```python
from build123d import *

# Parameters (mm, degrees)
F0_R     = 1.5
F1_DEPTH = 20
F2_W     = 3
F2_H     = 10
F3_DEPTH = 12


with BuildPart() as f1:
    # F0 (on Top) → F1 (new body)
    with BuildSketch(Plane.XY):
        with BuildLine():
            ThreePointArc((15, 2), (14.12132, 4.12132), (12, 5))
            Line((12, 5), (-12, 5))
            ThreePointArc((-12, 5), (-14.12132, 4.12132), (-15, 2))
            Line((-15, 2), (-15, -2))
            ThreePointArc((-15, -2), (-14.12132, -4.12132), (-12, -5))
            Line((-12, -5), (12, -5))
            ThreePointArc((12, -5), (14.12132, -4.12132), (15, -2))
            Line((15, -2), (15, 2))
        make_face()
        with Locations((-10, 0)):
            Circle(F0_R, mode=Mode.SUBTRACT)
        with Locations((10, 0)):
            Circle(F0_R, mode=Mode.SUBTRACT)
    extrude(amount=F1_DEPTH)

    # F2 (on face) → F3 (cut)
    with BuildSketch(Plane(origin=(0, 0, 0), x_dir=(1, 0, 0), z_dir=(0, 0, -1))):
        Rectangle(F2_W, F2_H)
    extrude(amount=-F3_DEPTH, mode=Mode.SUBTRACT)

    # F4: F1 across face


with BuildPart() as f1_1:
    add(f1.part)
    add(f1.part.mirror(Plane.XY.offset(20)))


solid = f1_1.part
```
For this review, take the finished solid that the model builds, in its own axes (mm). A direction names the side the tool comes from. Coordinates: 2 decimals unless noted, no trailing zeros. Order: outer loops, then holes, each group sorted by start corner. A loop starts at its lowest first (then second) coordinate and runs counter-clockwise, first axis right, second up. Notation, with made-up numbers: (31, 2.25) -> (90, 2.25) arc R7 cw to (90, 12.25) -> close; hole circle Ø7 at (-22, 21). An arc over 180 degrees is marked (long way). Use CSV: the item, a comma, the result in double quotes. Start each with the question number.
Item 1: We need section B-B, the plane x = -10. Give the boundary of the cut face in (y, z).
Item 2: Insertion check: pin 1 (3.5 mm diameter, centred on x = 10, y = 0, fed in from +Z); pin 2 (1.5 mm diameter, centred on x = -0.5, y = 0, fed in from -Z); pin 3 (0.9 mm diameter, centred on x = 0, y = 1, fed in from +Z). Each pin has a flat end and moves straight along its axis. Give the tip position at first contact, or say it passes through.
Item 3: Wall thickness on probe 1 along Y at (x, z) = (-10, 13); probe 2 along X at (y, z) = (-2, 32); probe 3 along Y at (x, z) = (-10.75, 33.5): over which ranges is each line inside the solid? List them lowest first.
Item 4: We need section D-D, the plane z = 16.5. Give the boundary of the cut face in (x, y), then the cut area to 3 significant figures.
Item 5: Draft analysis for pull direction Y (two halves, no side actions). For faces 1 (the face through (14.14, 4.1, 20.28)), 2 (the face through (-11.5, 0.07, 20.28)), 3 (the face through (8.5, 0.07, 20.28)), 4 (the face through (8, 0, 40)), state which applies: pulls with the +Y half, pulls with the -Y half, needs draft (parallel to the pull), parting line crosses it, or undercut.
Item 6: We need section C-C, the plane y = 0. Give the boundary of the cut face in (x, z), then the cut area to 3 significant figures.
Item 7: We need section A-A, the plane z = 10. Give the boundary of the cut face in (x, y), then the cut area to 3 significant figures.
Item 8: For faces 5 (the face through (-15, 0, 20)), 6 (the face through (1.5, 0, 6)), 7 (the face through (1.5, 0, 34)), list the 3-axis set-ups (+Z, -Z, +X, -X, +Y, -Y) from which the entire face can be reached by the end or side of a thin tool; tool diameter is ignored.
Derived:
1,outline,"(-5, 0) -> (-1.5, 0) -> (-1.5, 40) -> (-5, 40) -> close; (1.5, 0) -> (5, 0) -> (5, 40) -> (1.5, 40) -> close"
2,pin 1,"stops at z = 40"
2,pin 2,"stops at z = 12"
2,pin 3,"stops at z = 28"
3,probe 1,"y = -5 to -1.5, 1.5 to 5"
3,probe 2,"x = -15 to -1.5, 1.5 to 15"
3,probe 3,"y = -5 to -1.3, 1.3 to 5"
4,outline,"(-15, -2) arc R3 ccw to (-12, -5) -> (12, -5) arc R3 ccw to (15, -2) -> (15, 2) arc R3 ccw to (12, 5) -> (-12, 5) arc R3 ccw to (-15, 2) -> close; hole circle Ø3 at (-10, 0); hole circle Ø3 at (10, 0)"
4,area,"278 mm^2"
5,face 1,"pulls with the +Y half"
5,face 2,"undercut"
5,face 3,"undercut"
5,face 4,"needs draft"
6,outline,"(-15, 0) -> (-11.5, 0) -> (-11.5, 40) -> (-15, 40) -> close; (-8.5, 0) -> (-1.5, 0) -> (-1.5, 12) -> (1.5, 12) -> (1.5, 0) -> (8.5, 0) -> (8.5, 40) -> (1.5, 40) -> (1.5, 28) -> (-1.5, 28) -> (-1.5, 40) -> (-8.5, 40) -> close; (11.5, 0) -> (15, 0) -> (15, 40) -> (11.5, 40) -> close"
6,area,"888 mm^2"
7,outline,"(-15, -2) arc R3 ccw to (-12, -5) -> (-1.5, -5) -> (-1.5, 5) -> (-12, 5) arc R3 ccw to (-15, 2) -> close; (1.5, -5) -> (12, -5) arc R3 ccw to (15, -2) -> (15, 2) arc R3 ccw to (12, 5) -> (1.5, 5) -> close; hole circle Ø3 at (-10, 0); hole circle Ø3 at (10, 0)"
7,area,"248 mm^2"
8,face 5,"+Z, -Z, -X, +Y, -Y"
8,face 6,"-Z, +Y, -Y"
8,face 7,"+Z, +Y, -Y"
